Autodesk Inventor part; units mm, degrees
ref_plane "YZ Plane" through (0, 0, 0) normal (1, 0, 0) x (0, 1, 0)
ref_plane "XZ Plane" through (0, 0, 0) normal (0, 1, 0) x (-1, 0, 0)
ref_plane "XY Plane" through (0, 0, 0) normal (0, 0, 1) x (1, 0, 0)
sketch "Эскиз1" plane through (0, 0, 0) normal (0, 1, 0) x (-1, 0, 0)
  circle A0 centre (0, 0) radius 8.45
  circle A1 centre (0, 0) radius 9.45
  line L0 (0, 0) -> (7.5409, 5.6954)
  line L1 (0, 0) -> (7.5409, -5.6954)
  point P0 (6.7429, -5.0927)
  point P1 (6.7429, 5.0927)
  dimension "d0" = 16.9
  dimension "d1" = 18.9
extrude "Выдавливание1" add sketch "Эскиз1" along normal blind 30 contours A0 L1 A1 L0 picked at (6.7284, 6.0563)
sketch "Эскиз2" plane through (0, 30, 0) normal (0, 1, 0) x (1, 0, 0)
  arc A0 (-6.7429, -5.0927) -> (-7.6356, -4.5628) centre (-9.4442, -8.6266) ccw
  arc A1 (-7.6356, -4.5628) -> (-8.7926, -6.3685) centre (-8.07, -5.558) ccw
  line L0 (-8.7926, -6.3685) -> (-8.1213, -5.5141)
  arc A2 (-7.5423, -5.6808) -> (-8.1213, -5.5141) centre (-7.9107, -5.8712) ccw
  line L1 (-6.7429, -5.0927) -> (-7.5409, -5.6954)
  line L2 (-7.5409, -5.6954) -> (-6.7429, -5.0927)
  line L3 (-7.5409, -5.6954) -> (-7.5423, -5.6808)
  line L4 (-0.0151, 0) -> (-3.489, 0)
  arc A3 (-7.6356, 4.5628) -> (-6.7429, 5.0927) centre (-9.4442, 8.6266) ccw
  arc A4 (-8.1213, 5.5141) -> (-7.5423, 5.6808) centre (-7.9107, 5.8712) ccw
  line L5 (-6.7429, 5.0927) -> (-7.5409, 5.6954)
  line L6 (-7.5409, 5.6954) -> (-6.7429, 5.0927)
  line L7 (-7.5409, 5.6954) -> (-7.5423, 5.6808)
  arc A5 (-8.7926, 6.3685) -> (-7.6356, 4.5628) centre (-8.07, 5.558) ccw
  line L8 (-8.7926, 6.3685) -> (-8.1213, 5.5141)
  point P0 (-6.7429, 5.0927)
  point P1 (-5.3694, -4.0591)
  point P2 (-7.5409, 5.6954)
  point P3 (-5.3694, 4.0591)
  point P4 (-7.5409, 5.6954)
  dimension "d25" = 1.0859
sketch "Эскиз3" plane through (0, 30, 0) normal (0, 1, 0) x (1, 0, 0)
  arc A0 (-7.5409, -5.6954) -> (-7.5409, 5.6954) centre (0, 0) ccw
  line L0 (11.5, -6.95) -> (11.5, 6.95)
  arc A1 (-6.7429, -5.0927) -> (-6.7429, 5.0927) centre (0, 0) ccw
  arc A2 (0, -8.45) -> (0, 8.45) centre (0, 0) ccw
  line L1 (0, -9.45) -> (0, -8.45)
  line L2 (0, 8.45) -> (0, 9.45)
  line L3 (11.5, 6.95) -> (11.5, 10.95)
  line L4 (11.5, -6.95) -> (11.5, -10.95)
  line L5 (0, 4.95) -> (0, 9.45)
  line L6 (11.5, -10.95) -> (0, -10.95)
  line L7 (0, -10.95) -> (0, -9.45)
  line L8 (11.5, 10.95) -> (0, 10.95)
  line L9 (0, 10.95) -> (0, 9.45)
  point P0 (0, 8.45)
  dimension "d13" = 4
  dimension "d14" = 4
  dimension "d22" = 21.9
  dimension "d23" = 2.5
extrude "Выдавливание3" add sketch "Эскиз3" against normal blind 30
ref_plane "РабПлоскость1" through (11.5, 20, 4.95) normal (1, 0, 0) x (0, 0, -1)
sketch "Эскиз4" plane through (11.5, 20, 4.95) normal (1, 0, 0) x (0, 0, -1)
  line L0 (4.95, -20) -> (4.95, 10)
  line L1 (1, 10) -> (8.9, 10)
  circle A0 centre (4.95, -12) radius 5
  line L2 (14.4, -20) -> (-4.5, -20)
  circle A1 centre (4.95, 2) radius 5
  line L3 (-4.5, 10) -> (14.4, 10)
  point P0 (7.3306, 10)
  point P1 (2.5694, 10)
  point P2 (4.95, 10)
  dimension "d15" = 10
  dimension "d16" = 8
  dimension "d17" = 10
  dimension "d18" = 8
extrude "Выдавливание4" cut sketch "Эскиз4" against normal blind 2
extrude "Выдавливание5" add sketch "Эскиз2" against normal blind 30
properties part number "крепление маркера 17мм"
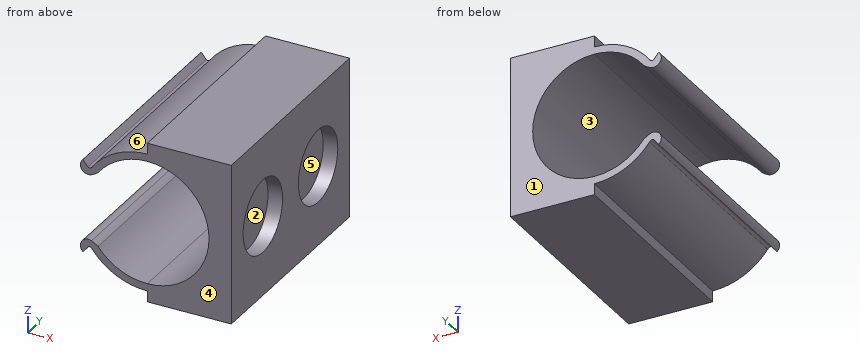
CAD build for the part. Positions are in the model's coordinates, mm. Face numbers are marked on the shaded views. A direction names the side the tool comes from. Coordinates: 2 decimals unless noted, no trailing zeros. Loops run counter-clockwise (first coordinate to the right, second up) from the corner with the lowest first, then second, coordinate; pieces in that order, holes last. Notation, with made-up numbers: (-9.75, -2) -> (36.25, -2) arc R10 cw to (36.25, 15) -> close; hole circle Ø6 at (45, -32.5). An arc over 180 degrees is marked (long way). One line per item, written item: value.
1. Slice it at C-C on z = 0. Write the cut outline in (x, y).
Answers:
outline: (8.45, 0) -> (11.5, 0) -> (11.5, 3) -> (9.5, 3) -> (9.5, 13) -> (11.5, 13) -> (11.5, 17) -> (9.5, 17) -> (9.5, 27) -> (11.5, 27) -> (11.5, 30) -> (8.45, 30) -> close
2. Pull direction Z, two halves, no side cores. Call the marked faces 4, 5 and 6: pulls with the +Z half, pulls with the -Z half, needs draft (parallel to the pull), parting line crosses it, or undercut.
Answers:
face 4: needs draft
face 5: undercut
face 6: pulls with the +Z half
3. Flat gauge pins, fed straight in: P1, Ø5, axis at y = 8.5, z = -6.5, coming from the -X side; P2, Ø9, axis at y = 8, z = 0, coming from the +X side; P3, Ø1.2, axis at y = 22, z = -10.5, coming from the -X side. Where does each tip first touch, or does it go through?
Answers:
P1: stops at x = -9.16
P2: stops at x = 9.5
P3: stops at x = 0
4. Drill centre lines: line 1 (Y direction, x = 10.15, z = 0); line 2 (Z direction, x = 10.8, y = 22); line 3 (X direction, y = 2.25, z = -6.25). Where is each one in solid material? Low to high. Write a range as [from, to].
Answers:
line 1: y = [0, 3], [13, 17], [27, 30]
line 2: z = [-10.95, -5], [5, 10.95]
line 3: x = [-8.91, -8.7], [-7.09, -5.69], [5.69, 11.5]
5. Slice it at A-A on z = -7.75. Write the cut outline in (x, y), and give its area (3 significant figures).
Answers:
outline: (-5.41, 0) -> (-3.37, 0) -> (-3.37, 30) -> (-5.41, 30) -> close; (3.37, 0) -> (11.5, 0) -> (11.5, 30) -> (3.37, 30) -> close
area: 305 mm^2
6. Which spindle directions (+Z, -Z, +X, -X, +Y, -Y) get a long thin tool onto all of the face, cutting with end or side? Do the marked faces 1, 2 and 3. Say none if no direction does.
Answers:
face 1: +Z, -Z, +X, -X, +Y
face 2: +X
face 3: +Y, -Y
7. Slice it at B-B on x = -3.25. Write the cut outline in (y, z), and give its area (3 significant figures).
Answers:
outline: (0, -8.87) -> (30, -8.87) -> (30, -7.8) -> (0, -7.8) -> close; (0, 7.8) -> (30, 7.8) -> (30, 8.87) -> (0, 8.87) -> close
area: 64.4 mm^2
